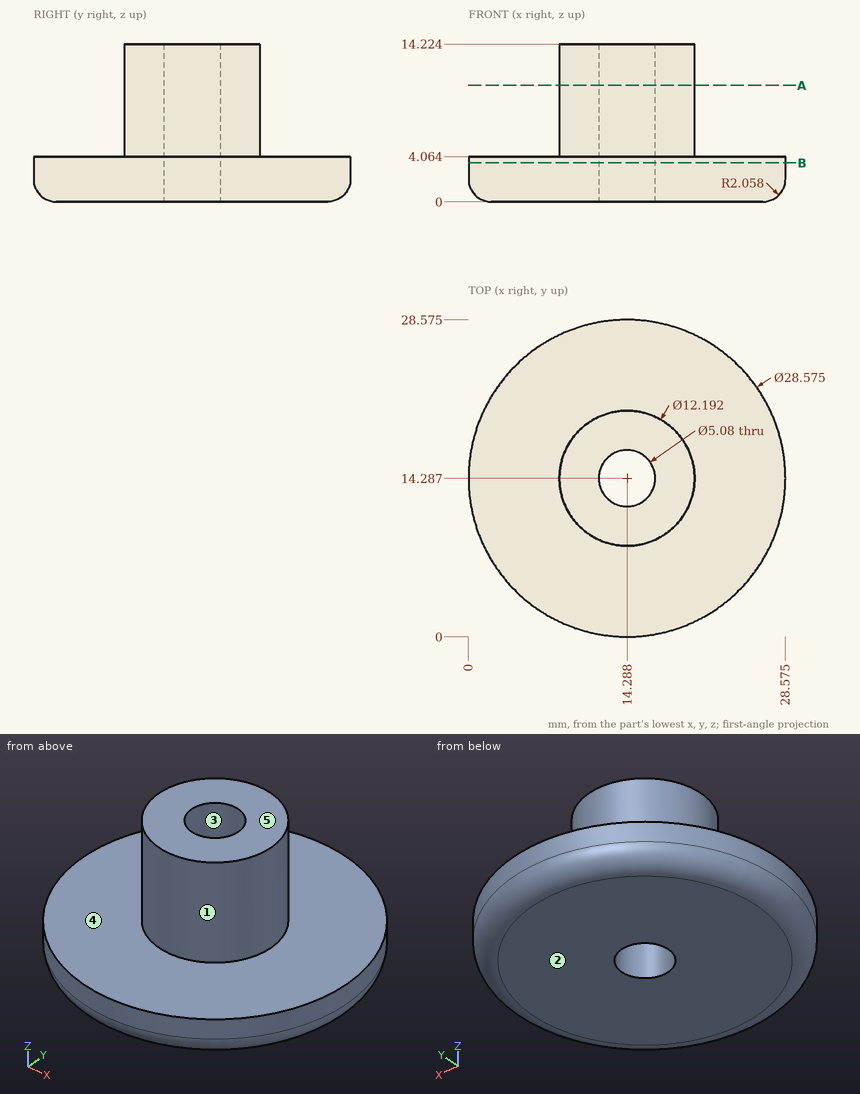
Can you work these out from the drawing? Everything is in mm from the part's minimum corner. A direction names the side the tool comes from. Round coordinates to 2 decimals unless told otherwise and drop trailing zeros. Loops run counter-clockwise (first coordinate to the right, second up) from the corner with the lowest first, then second, coordinate; pieces in that order, holes last.
1. If I drill on line 1 along Y through (x, z) = (14.25, 8.75); line 2 along Z through (x, y) = (11.5, 24.5) (1 decimal); line 3 along X through (y, z) = (14, 10.5) (1 decimal), over which ranges is the centre line in solid material (lowest first)?
Answer list:
line 1: y = 8.19 to 11.75, 16.83 to 20.38
line 2: z = 0 to 4.1
line 3: x = 8.2 to 11.8, 16.8 to 20.4
2. We'd pull the mould along Y, two halves only. Please class the marked faces 1, 2 and 3: +Y half, -Y half, draft (parallel to the pull), parting line (faces both ways), or undercut.
Answer list:
face 1: parting line
face 2: draft
face 3: undercut
3. If we section it at A-A on z = 10.5: Write out the boundary of the cut face in (x, y) (1 decimal).
Answer list:
outline: circle Ø12.2 at (14.3, 14.3); hole circle Ø5.1 at (14.3, 14.3)
4. If we section it at B-B on z = 3.5: Write out the boundary of the cut face in (x, y) (1 decimal), plus the area to 3 significant figures.
Answer list:
outline: circle Ø28.6 at (14.3, 14.3); hole circle Ø5.1 at (14.3, 14.3)
area: 621 mm2
5. For P1, Ø1.5, axis at x = 12, z = 9.5, coming from the -Y side; P2, Ø1.5, axis at x = 20, z = 5, coming from the +Y side; P3, Ø6, axis at x = 22.5, y = 4.5, coming from the +Z side, each with a flat end and sliding along its axis, tell me the tip position at first contact or that it passes through.
Answer list:
P1: stops at y = 8.39
P2: stops at y = 17.83
P3: stops at z = 4.06
6. Which directions (+Z, -Z, +X, -X, +Y, -Y) give clear straight access to the entire face, cutting with the end or side of a thin tool? Please do the marked faces 4 and 5.
Answer list:
face 4: +Z
face 5: +Z, +X, -X, +Y, -Y
